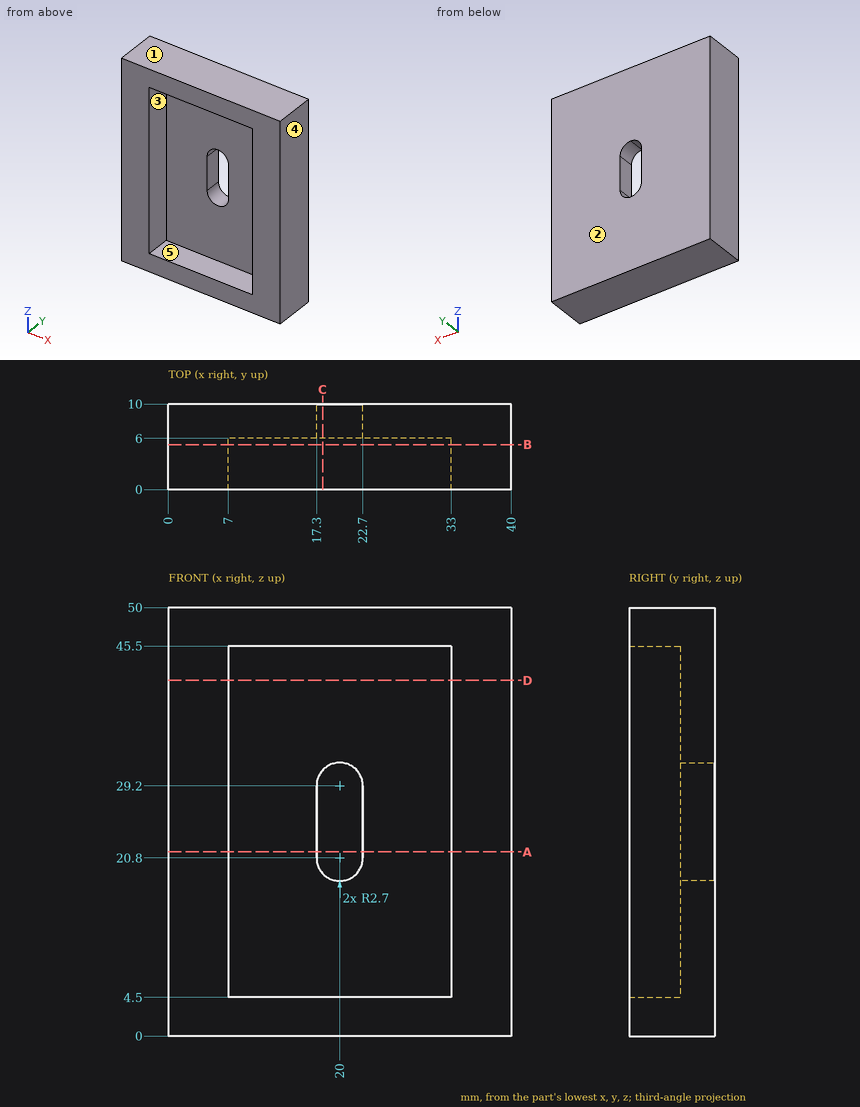
Check sheet for the drawn part. Datum: minimum x, y, z corner. Units: mm. A direction names the side the tool comes from. Round coordinates to 2 decimals unless told otherwise and drop trailing zeros. Write each loop counter-clockwise with the first axis right and the second up, starting at its lowest first coordinate (ties: lowest second). Pieces come first, ordered by that corner, then holes. Notation, with made-up numbers: (35.5, -39) - (81.5, -39) arc R8 ccw to (81.5, -31) - close; hole circle Ø9 at (-7.5, 14.25). An arc over 180 degrees is marked (long way). Return JSON: item names as keys, results as strings.
Q1. Access from +Z, -Z, +X, -X, +Y, -Y to the whole of each face (thin tool, end or side, straight path). Record for the marked faces 4 and 5.
Returned:
{"face 4": "+Z, -Z, +X, +Y, -Y", "face 5": "-Y"}
Q2. Cross-section at A-A (z = 21.5). Record the boundary of the cut face in (x, y), then the cut area to 3 significant figures.
Returned:
{"outline": "(0, 0) - (7, 0) - (7, 6) - (17.3, 6) - (17.3, 10) - (0, 10) - close; (22.7, 6) - (33, 6) - (33, 0) - (40, 0) - (40, 10) - (22.7, 10) - close", "area": "222 mm²"}
Q3. Scan lines: L1, parallel to Z at x = 14, y = 5.75; L2, parallel to X at y = 4.25, z = 8; L3, parallel to X at y = 8.5, z = 27. Record each from-to range of solid material in increasing order. Write a range as from..to.
Returned:
{"L1": "z = 0..4.5, 45.5..50", "L2": "x = 0..7, 33..40", "L3": "x = 0..17.3, 22.7..40"}
Q4. Cross-section at C-C (x = 18). Record the boundary of the cut face in (y, z).
Returned:
{"outline": "(0, 0) - (10, 0) - (10, 18.99) - (6, 18.99) - (6, 4.5) - (0, 4.5) - close; (0, 45.5) - (6, 45.5) - (6, 31.01) - (10, 31.01) - (10, 50) - (0, 50) - close"}
Q5. Cross-section at D-D (z = 41.5). Record the boundary of the cut face in (x, y).
Returned:
{"outline": "(0, 0) - (7, 0) - (7, 6) - (33, 6) - (33, 0) - (40, 0) - (40, 10) - (0, 10) - close"}
Q6. Draft check along Z on the marked faces 1, 2 and 3. Enter one of: released by +Z, released by -Z, zero draft, split by the parting line, or undercut.
Returned:
{"face 1": "released by +Z", "face 2": "zero draft", "face 3": "undercut"}
Q7. Cross-section at B-B (y = 5.25). Record the boundary of the cut face in (x, z), then the cut area to 3 significant figures.
Returned:
{"outline": "(0, 0) - (40, 0) - (40, 50) - (0, 50) - close; hole (7, 4.5) - (33, 4.5) - (33, 45.5) - (7, 45.5) - close", "area": "934 mm²"}
